```python
from build123d import *

# Parameters (mm, degrees)
SKETCH_W        = 33.2
SKETCH_H        = 7
SKETCH_R        = 1.6
PAD_DEPTH       = 25
SKETCH001_R     = 1.6
PAD001_DEPTH    = 25
FILLET_R        = 4.99
SKETCH002_W     = 10
SKETCH002_H     = 7.5
POCKET_DEPTH    = 33.201
POCKET001_DEPTH = 2.5
FILLET001_R     = 3


with BuildPart() as part:
    # Sketch → Pad (new body)
    with BuildSketch(Plane.XY):
        Rectangle(SKETCH_W, SKETCH_H)
        with Locations((-13, 0)):
            Circle(SKETCH_R, mode=Mode.SUBTRACT)
        with Locations((13, 0)):
            Circle(SKETCH_R, mode=Mode.SUBTRACT)
    extrude(amount=PAD_DEPTH)

    # Sketch001 (on Face8 of Pad) → Pad001 (join)
    with BuildSketch(Plane.XY.offset(25)):
        with BuildLine():
            ThreePointArc((5, 8.5), (0, 13.5), (-5, 8.5))
            Line((-5, 8.5), (-5, 3.5))
            Line((-5, 3.5), (5, 3.5))
            Line((5, 3.5), (5, 8.5))
        make_face()
        with Locations((0, 8.5)):
            Circle(SKETCH001_R, mode=Mode.SUBTRACT)
    extrude(amount=-PAD001_DEPTH)

    # Fillet
    fillet_edges = [part.edges().sort_by_distance(p)[0] for p in [
        (-5, 3.5, 12.5),
        (5, 3.5, 12.5),
    ]]
    fillet(fillet_edges, radius=FILLET_R)

    # Sketch002 (on Face4 of Fillet) → Pocket (cut, through all)
    with BuildSketch(Plane(origin=(-16.6, 0, 0), x_dir=(0, -1, 0), z_dir=(-1, 0, 0))):
        with Locations((-8.5, 12.5)):
            Rectangle(SKETCH002_W, SKETCH002_H)
    extrude(amount=-POCKET_DEPTH, mode=Mode.SUBTRACT)

    # Sketch004 (on Face6 of Pocket) → Pocket001 (cut)
    with BuildSketch(Plane(origin=(0, 0, 0), x_dir=(1, 0, 0), z_dir=(0, 0, -1))):
        Polygon((2.8, -6.883419), (0, -5.266838), (-2.8, -6.883419), (-2.8, -10.116581), (0, -11.733162), (2.8, -10.116581), align=None)
    extrude(amount=-POCKET001_DEPTH, mode=Mode.SUBTRACT)

    # Fillet001
    fillet001_edges = [part.edges().sort_by_distance(p)[0] for p in [
        (16.6, 3.5, 4.375),
        (16.6, -3.5, 12.5),
        (-16.6, 3.5, 20.625),
        (-16.6, -3.5, 12.5),
    ]]
    fillet(fillet001_edges, radius=FILLET001_R)


solid = part.part
```
Verification items for the finished model (mm, model axes). A direction names the side the tool comes from. Give positions to 0.01 mm unless a question says otherwise; leave off trailing zeros. Order: outer loops, then holes, each group sorted by start corner. A loop starts at its lowest first (then second) coordinate and runs counter-clockwise, first axis right, second up. Notation, with made-up numbers: M 85,-0.5 L 91,-0.5 A24 ccw 91,30.5 Z; hole C 66.25,20 d4. An arc over 180 degrees is marked long. Answer in a Markdown table with one row per item. Add a question column.
Item 1: Mould release check, pull along X, two halves, no side actions. Record for faces 4 (the cylindrical face through (15.74, -2.6, 12.68)), 5 (the flat face through (-1.42, 10.914, 1.232)), 6 (the flat face through (0, 1, 0)): released by +X, released by -X, zero draft, split by the parting line, or undercut.
Item 2: Gauge pin test, flat ends, axial feed: pin 1 (1.2 mm diameter, centred on y = 8.5, z = 1, fed in from -X) (3 decimals); pin 2 (1.7 mm diameter, centred on x = 0.5, y = 8, fed in from -Z); pin 3 (1.2 mm diameter, centred on y = 8.5, z = 2, fed in from +X) (3 decimals); pin 4 (6 mm diameter, centred on y = 4, z = 20, fed in from +X). Record the tip position at first contact, or that the pin passes through.
Item 3: Section check A-A, the plane x = 13. Enter the section's corners in (y, z).
Item 4: Scan lines: probe 1 along Y at (x, z) = (13, 12.25); probe 2 along Z at (x, y) = (2, 6.25); probe 3 along X at (y, z) = (-1.25, 18). Record each from-to range of solid material in increasing order. Write a range as from..to.
Item 5: Section check D-D, the plane z = 20. State how many separate pieces and enclosed holes the cut face has, and give its area (3 significant figures).
Item 6: Section check B-B, the plane z = 15.5. Enter the section's corners in (x, y), and give its area (3 significant figures).
Item 7: Tool access check on faces 1 (the flat face through (-1.38, 6.064, 1.232)), 2 (the flat face through (0, 6, 16.25)), 3 (the flat face through (0, -3.5, 12)). Record the directions out of +Z, -Z, +X, -X, +Y, -Y that give a thin tool (end or side, any length) a straight path to the whole face; none if there is none.
Item 8: Section check C-C, the plane x = 1. Enter the section's corners in (y, z), and give its area (3 significant figures).
Filled sheet:
| question | item | result |
|---|---|---|
| 1 | face 4 | released by +X |
| 1 | face 5 | undercut |
| 1 | face 6 | zero draft |
| 2 | pin 1 | stops at x = -5.035 |
| 2 | pin 2 | passes through |
| 2 | pin 3 | stops at x = 5.035 |
| 2 | pin 4 | stops at x = 16.56 |
| 3 | outline | M -3.5,0 L -1.6,0 L -1.6,25 L -3.5,25 Z; M 1.6,0 L 3.5,0 L 3.5,25 L 1.6,25 Z |
| 4 | probe 1 | y = -3.5..-1.6, 1.6..3.5 |
| 4 | probe 2 | z = 0..8.75, 16.25..25 |
| 4 | probe 3 | x = -16.5..-14, -12..12, 14..16.5 |
| 5 | separate pieces | 1 |
| 5 | enclosed holes | 3 |
| 5 | area | 301 mm^2 |
| 6 | outline | M -16.6,-0.5 A3 ccw -13.6,-3.5 L 13.6,-3.5 A3 ccw 16.6,-0.5 L 16.6,0.5 A3 ccw 13.6,3.5 L -13.6,3.5 A3 ccw -16.6,0.5 Z; hole C -13,0 d3.2; hole C 13,0 d3.2 |
| 6 | area | 209 mm^2 |
| 7 | face 1 | -Z |
| 7 | face 2 | +X, -X, +Y |
| 7 | face 3 | +Z, -Z, +X, -X, -Y |
| 8 | outline | M -3.5,0 L 5.84,0 L 5.84,2.5 L 7.25,2.5 L 7.25,8.75 L 3.5,8.75 L 3.5,16.25 L 7.25,16.25 L 7.25,25 L -3.5,25 Z; M 9.75,2.5 L 11.16,2.5 L 11.16,0 L 13.4,0 L 13.4,8.75 L 9.75,8.75 Z; M 9.75,16.25 L 13.4,16.25 L 13.4,25 L 9.75,25 Z |
| 8 | area | 297 mm^2 |
